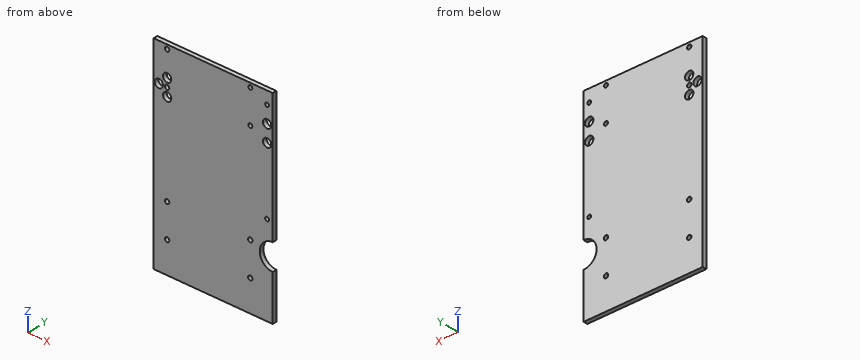
from build123d import *

# Parameters (mm, degrees)
SKETCH1_R           = 1.85
SKETCH1_R_2         = 1.905
SKETCH1_R_3         = 2.1
SKETCH1_R_4         = 4
BOSS_EXTRUDE1_DEPTH = 4


with BuildPart() as part:
    # Sketch1 → Boss-Extrude1 (new body)
    with BuildSketch(Plane(origin=(0, 0, 0), x_dir=(1, 0, 0), z_dir=(0, 1, 0))):
        with BuildLine():
            Line((-141, -139.759258716), (-26.44, -139.759258716))
            Line((-26.44, -139.759258716), (-26.44, -14.400783004))
            ThreePointArc((-26.44, -14.400783004), (-38.907528285, -1.933254719), (-26.44, 10.534273565))
            Line((-26.44, 10.534273565), (-26.44, 54.240741284))
            Line((-26.44, 54.240741284), (-141, 54.240741284))
            Line((-141, 54.240741284), (-141, -139.759258716))
        make_face()
        with Locations((-31.84, -31.759258716)):
            Circle(SKETCH1_R, mode=Mode.SUBTRACT)
        with Locations((-31.84, -127.759258716)):
            Circle(SKETCH1_R, mode=Mode.SUBTRACT)
        with Locations((-48, -135.759258716)):
            Circle(SKETCH1_R_2, mode=Mode.SUBTRACT)
        with Locations((-48, -103.759258716)):
            Circle(SKETCH1_R_2, mode=Mode.SUBTRACT)
        with Locations((-128, -135.759258716)):
            Circle(SKETCH1_R_3, mode=Mode.SUBTRACT)
        with Locations((-128, -103.759258716)):
            Circle(SKETCH1_R_3, mode=Mode.SUBTRACT)
        with Locations((-136, -103.759258716)):
            Circle(SKETCH1_R_4, mode=Mode.SUBTRACT)
        with Locations((-128, -95.759258716)):
            Circle(SKETCH1_R_4, mode=Mode.SUBTRACT)
        with Locations((-128, -111.759258716)):
            Circle(SKETCH1_R_4, mode=Mode.SUBTRACT)
        with Locations((-128, -7.759258716)):
            Circle(SKETCH1_R_3, mode=Mode.SUBTRACT)
        with Locations((-128, 24.240741284)):
            Circle(SKETCH1_R_3, mode=Mode.SUBTRACT)
        with Locations((-48, -7.759258716)):
            Circle(SKETCH1_R_3, mode=Mode.SUBTRACT)
        with Locations((-48, 24.240741284)):
            Circle(SKETCH1_R_3, mode=Mode.SUBTRACT)
        with Locations((-31.84, -111.759258716)):
            Circle(SKETCH1_R_4, mode=Mode.SUBTRACT)
        with Locations((-31.84, -95.759258716)):
            Circle(SKETCH1_R_4, mode=Mode.SUBTRACT)
    extrude(amount=-BOSS_EXTRUDE1_DEPTH)


solid = part.part
Here's how the part is built. I have some questions about the finished solid (model axes, mm). Round coordinates to 2 decimals unless told otherwise and drop trailing zeros. Loops run counter-clockwise (first coordinate to the right, second up) from the corner with the lowest first, then second, coordinate; pieces in that order, holes last. Notation, with made-up numbers: (-14, 35) - (10, 35) arc R12 cw to (10, 58) - close; hole circle Ø2 at (-18, 87). An arc over 180 degrees is marked (long way). One line per question, with ' | ' between items. Start each with the question number.
Q1. I want a section at C-C (y = -2.2). State how many separate pieces and enclosed holes the cut face has, then the cut area to 3 significant figures.
Q2. I want a section at B-B (x = -48). Write out the boundary of the cut face in (y, z), then the cut area to 3 significant figures.
Q3. Will this pin go through, and if not, where does the flat tip stop? pin 1 (2.5 mm diameter, centred on x = -128, z = -24.24, fed in from -Y).
Q4. I want a section at D-D (x = -31.84). Write out the boundary of the cut face in (y, z).
Q5. I want a section at A-A (x = -136). Write out the boundary of the cut face in (y, z).
Q6. Please list where these lines run through material, in increasing order: line 1 (Z direction, x = -48, y = -2.1); line 2 (X direction, y = -0.4, z = 114); line 3 (X direction, y = -1.7, z = 103). Write a range as [from, to].
Response values:
1) separate pieces: 1 | enclosed holes: 15 | area: 21,600 mm²
2) outline: (-4, -54.24) - (0, -54.24) - (0, -26.34) - (-4, -26.34) - close; (-4, -22.14) - (0, -22.14) - (0, 5.66) - (-4, 5.66) - close; (-4, 9.86) - (0, 9.86) - (0, 101.85) - (-4, 101.85) - close; (-4, 105.66) - (0, 105.66) - (0, 133.85) - (-4, 133.85) - close; (-4, 137.66) - (0, 137.66) - (0, 139.76) - (-4, 139.76) - close | area: 712 mm²
3) pin 1: passes through
4) outline: (-4, -54.24) - (0, -54.24) - (0, -9.3) - (-4, -9.3) - close; (-4, 13.17) - (0, 13.17) - (0, 29.91) - (-4, 29.91) - close; (-4, 33.61) - (0, 33.61) - (0, 91.76) - (-4, 91.76) - close; (-4, 99.76) - (0, 99.76) - (0, 107.76) - (-4, 107.76) - close; (-4, 115.76) - (0, 115.76) - (0, 125.91) - (-4, 125.91) - close; (-4, 129.61) - (0, 129.61) - (0, 139.76) - (-4, 139.76) - close
5) outline: (-4, -54.24) - (0, -54.24) - (0, 99.76) - (-4, 99.76) - close; (-4, 107.76) - (0, 107.76) - (0, 139.76) - (-4, 139.76) - close
6) line 1: z = [-54.24, -26.34], [-22.14, 5.66], [9.86, 101.85], [105.66, 133.85], [137.66, 139.76] | line 2: x = [-141, -131.31], [-124.69, -35.15], [-28.53, -26.44] | line 3: x = [-141, -139.93], [-132.07, -129.96], [-126.04, -49.75], [-46.25, -26.44]
